Here's how the part is built. I have some questions about the finished solid (model axes, mm). A direction names the side the tool comes from. Give positions to 0.01 mm unless a question says otherwise; leave off trailing zeros. Loops run counter-clockwise (first coordinate to the right, second up) from the corner with the lowest first, then second, coordinate; pieces in that order, holes last. Notation, with made-up numbers: (-33.75, -6.75) - (22.25, -6.75) arc R20 ccw to (22.25, 19.25) - close; hole circle Ø10 at (-30, 27.5). An arc over 180 degrees is marked (long way). Use a Markdown table: item, result.
from build123d import *

# Parameters (mm, degrees)
CROQUIS2_W              = 500
CROQUIS2_H              = 500
SALIENTE_EXTRUIR1_DEPTH = 100
CROQUIS3_R              = 150
SALIENTE_EXTRUIR2_DEPTH = 1000
CROQUIS5_R              = 75
SALIENTE_EXTRUIR4_DEPTH = 200


with BuildPart() as part:
    # Croquis2 → Saliente-Extruir1 (new body)
    with BuildSketch(Plane(origin=(0, 0, 0), x_dir=(1, 0, 0), z_dir=(0, 1, 0))):
        Rectangle(CROQUIS2_W, CROQUIS2_H)
    extrude(amount=SALIENTE_EXTRUIR1_DEPTH)

    # Croquis3 → Saliente-Extruir2 (add)
    with BuildSketch(Plane(origin=(0, 100, 0), x_dir=(1, 0, 0), z_dir=(0, 1, 0))):
        with Locations(Location((0, 0, 0), (0, 0, 270))):
            Circle(CROQUIS3_R)
    extrude(amount=SALIENTE_EXTRUIR2_DEPTH)

    # Croquis5 → Saliente-Extruir4 (add)
    with BuildSketch(Plane(origin=(0, 0, 0), x_dir=(0, 0, -1), z_dir=(1, 0, 0))):
        with Locations(Location((0, 969.265591665, 0), (0, 0, 180))):
            Circle(CROQUIS5_R)
    extrude(amount=SALIENTE_EXTRUIR4_DEPTH)


solid = part.part
(1) On a 3-axis mill with a long thin cutter (end or side, diameter ignored), from which of +Z, -Z, +X, -X, +Y, -Y can I reach the whole of each face in a straight line? I mean faces 1 (the face through (-3, 49, 250)), 2 (the face through (200, 968, -1)). Say none if no direction works.
A:
| item | result |
|---|---|
| face 1 | +Z, +X, -X, +Y, -Y |
| face 2 | +Z, -Z, +X, +Y |
(2) Suppose I cut it at B-B on x = 0. Write out the boundary of the cut face in (y, z).
A:
| item | result |
|---|---|
| outline | (0, -250) - (100, -250) - (100, -150) - (1100, -150) - (1100, 150) - (100, 150) - (100, 250) - (0, 250) - close |
(3) Will these pins go through, and if not, where does the flat tip stop? pin 1 (3 mm diameter, centred on x = -119.5, z = 115, fed in from -Y); pin 2 (1.5 mm diameter, centred on x = 134.5, y = 545.5, fed in from -Z); pin 3 (8 mm diameter, centred on y = 434, z = -43.5, fed in from -X); pin 4 (10 mm diameter, centred on x = -137, y = 681, fed in from +Z).
A:
| item | result |
|---|---|
| pin 1 | y = 0 |
| pin 2 | z = -67.9 |
| pin 3 | x = -144.71 |
| pin 4 | z = 71.25 |
(4) Suppose I cut it at D-D on z = 133. Write out the boundary of the cut face in (x, y), plus the area to 3 significant figures.
A:
| item | result |
|---|---|
| outline | (-250, 0) - (250, 0) - (250, 100) - (69.36, 100) - (69.36, 1100) - (-69.36, 1100) - (-69.36, 100) - (-250, 100) - close |
| area | 189,000 mm2 |
(5) Suppose I cut it at A-A on z = 0. Write out the boundary of the cut face in (x, y), plus the area to 4 significant figures.
A:
| item | result |
|---|---|
| outline | (-250, 0) - (250, 0) - (250, 100) - (150, 100) - (150, 894.27) - (200, 894.27) - (200, 1044.27) - (150, 1044.27) - (150, 1100) - (-150, 1100) - (-150, 100) - (-250, 100) - close |
| area | 357,500 mm2 |
(6) We'd pull the mould along Y, two halves only. Please class faces 3 (the face through (172.25, 997.99, 69.28)), 4 (the face through (-250, 49, 3)), 5 (the face through (-3, 0, -4)): pulls with the +Y half, pulls with the -Y half, needs draft (parallel to the pull), parting line crosses it, or undercut.
A:
| item | result |
|---|---|
| face 3 | undercut |
| face 4 | needs draft |
| face 5 | pulls with the -Y half |
(7) If I drill on line 1 (Z direction, x = -5.5, y = 241.5); line 2 (Y direction, x = -213.5, z = -174.5); line 3 (Y direction, x = 172, z = 47.5), over which ranges is the centre line in solid material (lowest first)?
A:
| item | result |
|---|---|
| line 1 | -149.9 to 149.9 |
| line 2 | 0 to 100 |
| line 3 | 0 to 100, 911.22 to 1027.31 |
(8) Suppose I cut it at C-C on y = 192. Write out the boundary of the cut face in (x, z), plus the area to 3 significant figures.
A:
| item | result |
|---|---|
| outline | circle Ø300 at (0, 0) |
| area | 70,700 mm2 |
